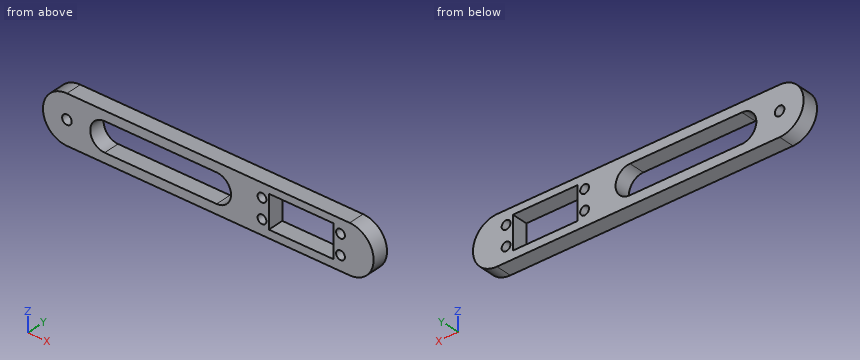
from build123d import *

# Parameters (mm, degrees)
SKETCH2_R           = 1.45
BOSS_EXTRUDE3_DEPTH = 10
SKETCH10_W          = 7.047144721
SKETCH10_H          = 19.860135122
BOSS_EXTRUDE7_DEPTH = 10
SKETCH12_R          = 1.45
BOSS_EXTRUDE8_DEPTH = 10
SKETCH13_R          = 2.925
CUT_EXTRUDE8_DEPTH  = 2
CUT_EXTRUDE9_DEPTH  = 10
SKETCH16_R          = 3
CUT_EXTRUDE10_DEPTH = 10
SKETCH6_R           = 2.75
SKETCH6_W           = 40.5
SKETCH6_H           = 20.5
CUT_EXTRUDE11_DEPTH = 10
SKETCH17_R          = 2.75
CUT_EXTRUDE12_DEPTH = 10


with BuildPart() as part:
    # Sketch2 → Boss-Extrude3 (new body)
    with BuildSketch(Plane(origin=(0, 0, 0), x_dir=(1, 0, 0), z_dir=(0, 1, 0))):
        with BuildLine():
            Line((0, 15), (100, 15))
            ThreePointArc((100, 15), (115, 0), (100, -15))
            Line((100, -15), (0, -15))
            ThreePointArc((0, -15), (-15, 0), (0, 15))
        make_face()
        with Locations(Location((0, 0, 0), (0, 0, 270))):
            Circle(SKETCH2_R, mode=Mode.SUBTRACT)
    extrude(amount=BOSS_EXTRUDE3_DEPTH)

    # Sketch10 → Boss-Extrude7 (add)
    with BuildSketch(Plane(origin=(0, 10, 0), x_dir=(1, 0, 0), z_dir=(0, 1, 0))):
        with Locations((94.781401452, 0.828180391)):
            Rectangle(SKETCH10_W, SKETCH10_H)
    extrude(amount=-BOSS_EXTRUDE7_DEPTH)

    # Sketch12 → Boss-Extrude8 (add)
    with BuildSketch(Plane(origin=(0, 10, 0), x_dir=(1, 0, 0), z_dir=(0, 1, 0))):
        with BuildLine():
            Line((-76.756351439, 15), (12.176052336, 15))
            ThreePointArc((12.176052336, 15), (27.176052336, 0), (12.176052336, -15))
            Line((12.176052336, -15), (-76.756351439, -15))
            ThreePointArc((-76.756351439, -15), (-91.756351439, 0), (-76.756351439, 15))
        make_face()
        with Locations(Location((-76.756351439, 0, 0), (0, 0, 270))):
            Circle(SKETCH12_R, mode=Mode.SUBTRACT)
    extrude(amount=-BOSS_EXTRUDE8_DEPTH)

    # Sketch13 → Cut-Extrude8 (cut)
    with BuildSketch(Plane(origin=(0, 10, 0), x_dir=(1, 0, 0), z_dir=(0, 1, 0))):
        with Locations(Location((-76.756351439, 0, 0), (0, 0, 270))):
            Circle(SKETCH13_R)
    extrude(amount=-CUT_EXTRUDE8_DEPTH, mode=Mode.SUBTRACT)

    # Sketch15 → Cut-Extrude9 (cut)
    with BuildSketch(Plane(origin=(0, 10, 0), x_dir=(1, 0, 0), z_dir=(0, 1, 0))):
        with BuildLine():
            Line((-53.180879761, 9.018176556), (16.819120239, 9.018176556))
            ThreePointArc((16.819120239, 9.018176556), (25.837296795, 0), (16.819120239, -9.018176556))
            Line((16.819120239, -9.018176556), (-53.180879761, -9.018176556))
            ThreePointArc((-53.180879761, -9.018176556), (-62.199056317, 0), (-53.180879761, 9.018176556))
        make_face()
    extrude(amount=-CUT_EXTRUDE9_DEPTH, mode=Mode.SUBTRACT)

    # Sketch16 → Cut-Extrude10 (cut)
    with BuildSketch(Plane(origin=(0, 10, 0), x_dir=(1, 0, 0), z_dir=(0, 1, 0))):
        with Locations(Location((-76.756351439, 0, 0), (0, 0, 270))):
            Circle(SKETCH16_R)
    extrude(amount=-CUT_EXTRUDE10_DEPTH, mode=Mode.SUBTRACT)

    # Sketch6 → Cut-Extrude11 (cut)
    with BuildSketch(Plane(origin=(0, 10, 0), x_dir=(1, 0, 0), z_dir=(0, 1, 0))):
        with Locations(Location((94.301250031, 5.9, 0), (0, 0, 270))):
            Circle(SKETCH6_R)
        with Locations(Location((94.301250031, -6.4, 0), (0, 0, 270))):
            Circle(SKETCH6_R)
        with Locations((69.751250031, -0.25)):
            Rectangle(SKETCH6_W, SKETCH6_H)
    extrude(amount=-CUT_EXTRUDE11_DEPTH, mode=Mode.SUBTRACT)

    # Sketch17 → Cut-Extrude12 (cut)
    with BuildSketch(Plane(origin=(0, 10, 0), x_dir=(1, 0, 0), z_dir=(0, 1, 0))):
        with Locations(Location((45.201250031, 5.9, 0), (0, 0, 270))):
            Circle(SKETCH17_R)
        with Locations(Location((45.201250031, -6.4, 0), (0, 0, 270))):
            Circle(SKETCH17_R)
    extrude(amount=-CUT_EXTRUDE12_DEPTH, mode=Mode.SUBTRACT)


solid = part.part
Can you work these out from the model? Positions are in its coordinate system, mm. Give positions to 0.01 mm unless a question says otherwise; leave off trailing zeros. Order: outer loops, then holes, each group sorted by start corner. A loop starts at its lowest first (then second) coordinate and runs counter-clockwise, first axis right, second up. Notation, with made-up numbers: M -7.5,70.25 L 25.5,70.25 A14 cw 25.5,77.25 Z; hole C 30.25,60.5 d3. An arc over 180 degrees is marked long. Use a Markdown table: item, result. Add a question column.
Item 1: Suppose I cut it at D-D (x = 82.5). List the corners of the cut face in (y, z) for me.
Item 2: If I drill on L1, parallel to X at y = 5, z = 0; L2, parallel to Z at x = -14.5, y = 4; L3, parallel to X at y = 6.5, z = 8, over which ranges is the centre line in solid material (lowest first)? Write a range as [from, to].
Item 3: Suppose I cut it at B-B (x = -11). List the corners of the cut face in (y, z) for me, then the cut area to 3 significant figures.
Item 4: Suppose I cut it at C-C (y = 3). List the corners of the cut face in (x, z) for me.
Item 5: Will these pins go through, and if not, where does the flat tip stop? pin 1 (4.5 mm diameter, centred on x = 45.2, z = 6.4, fed in from -Y); pin 2 (1.5 mm diameter, centred on y = 6, z = 6.5, fed in from +X); pin 3 (1.5 mm diameter, centred on y = 3.5, z = -2.5, fed in from -X).
Item 6: Suppose I cut it at A-A (z = 0). List the corners of the cut face in (x, y) for me, then the cut area to 3 significant figures.
Answer sheet:
| question | item | result |
|---|---|---|
| 1 | outline | M 0,-15 L 10,-15 L 10,-10 L 0,-10 Z; M 0,10.5 L 10,10.5 L 10,15 L 0,15 Z |
| 2 | L1 | x = [-91.76, -79.76], [-73.76, -62.2], [25.84, 49.5], [90, 115] |
| 2 | L2 | z = [-15, -9.02], [9.02, 15] |
| 2 | L3 | x = [-89.44, -57.34], [20.98, 42.96], [47.44, 49.5], [90, 92.06], [96.54, 112.69] |
| 3 | outline | M 0,-15 L 10,-15 L 10,-9.02 L 0,-9.02 Z; M 0,9.02 L 10,9.02 L 10,15 L 0,15 Z |
| 3 | area | 120 mm² |
| 4 | outline | M -76.76,-15 L 100,-15 A15 ccw 100,15 L -76.76,15 A15 ccw Z; hole C -76.76,0 d6; hole M -53.18,-9.02 L 16.82,-9.02 A9.02 ccw 16.82,9.02 L -53.18,9.02 A9.02 ccw Z; hole C 45.2,-5.9 d5.5; hole C 45.2,6.4 d5.5; hole M 49.5,-10 L 90,-10 L 90,10.5 L 49.5,10.5 Z; hole C 94.3,-5.9 d5.5; hole C 94.3,6.4 d5.5 |
| 5 | pin 1 | passes through |
| 5 | pin 2 | stops at x = 113.85 |
| 5 | pin 3 | stops at x = -91.65 |
| 6 | outline | M -91.76,0 L -79.76,0 L -79.76,10 L -91.76,10 Z; M -73.76,0 L -62.2,0 L -62.2,10 L -73.76,10 Z; M 25.84,0 L 49.5,0 L 49.5,10 L 25.84,10 Z; M 90,0 L 115,0 L 115,10 L 90,10 Z |
| 6 | area | 722 mm² |
